```python
from build123d import *

# Parameters (mm, degrees)
F0_W     = 26.5
F0_H     = 53
F1_DEPTH = 11
F2_R     = 5.75
F3_DEPTH = 120
F4_W     = 18
F4_H     = 11
F5_DEPTH = 25


with BuildPart() as f1:
    # F0 (on Top) → F1 (new body)
    with BuildSketch(Plane.XY):
        Rectangle(F0_W, F0_H)
    extrude(amount=F1_DEPTH)

    # F2 (on face) → F3 (join)
    with BuildSketch(Plane(origin=(0, 26.5, 0), x_dir=(-1, 0, 0), z_dir=(0, 1, 0))):
        with Locations((-5.25, 5.5)):
            Circle(F2_R)
    extrude(amount=F3_DEPTH)

    # F4 (on face) → F5 (join)
    with BuildSketch(Plane.XZ.offset(26.5)):
        with Locations((0, 5.5)):
            Rectangle(F4_W, F4_H)
    extrude(amount=F5_DEPTH)


solid = f1.part
```
Design review of the part built by this model. Coordinates are the model's own, in mm. A direction names the side the tool comes from. Round coordinates to 2 decimals unless told otherwise and drop trailing zeros. Write each loop counter-clockwise with the first axis right and the second up, starting at its lowest first coordinate (ties: lowest second). Pieces come first, ordered by that corner, then holes. Notation, with made-up numbers: (48, -18.5) -> (58, -18.5) arc R24 cw to (58, 12.5) -> close; hole circle Ø6 at (-27, 22). An arc over 180 degrees is marked (long way). Write item = value, one per line. Start each with the question number.
1) Wall thickness on probe 1 along X at (y, z) = (111.5, 6); probe 2 along Z at (x, y) = (-1.25, -27.5); probe 3 along Y at (x, z) = (-2.25, 9): over which ranges is each line inside the solid? List them lowest first. Write a range as from..to.
2) Take a section at A-A, the plane z = 5.5. State the section outline as (x, y) points.
3) Take a section at D-D, the plane x = -5. State the section outline as (y, z) points, plus the area to 3 significant figures.
4) Take a section at C-C, the plane y = -33. State the section outline as (x, z) points, plus the area to 3 significant figures.
5) Take a section at B-B, the plane x = 5.25. State the section outline as (y, z) points, plus the area to 3 significant figures.
6) Clearance check with flat-ended pins moving along their axes: pin 1 (1 mm diameter, centred on x = 10, y = 39, fed in from -Z); pin 2 (3 mm diameter, centred on x = 2.5, y = 36, fed in from -Z); pin 3 (5.5 mm diameter, centred on y = -37.5, z = 5, fed in from +X). State where each tip first meets the part, or that it passes through.
7) Tool access review of faces 1 (the face through (6, 85.7, 11.2)), 2 (the face through (-11, -26.5, 5)), 3 (the face through (11, -26.5, 5)): name each direction out of +Z, -Z, +X, -X, +Y, -Y from which nothing blocks a thin tool from reaching the whole face with its end or side.
Results list:
q1.probe_1 = -0.48..10.98
q1.probe_2 = 0..11
q1.probe_3 = -51.5..26.5
q2.outline = (-13.25, -26.5) -> (-9, -26.5) -> (-9, -51.5) -> (9, -51.5) -> (9, -26.5) -> (13.25, -26.5) -> (13.25, 26.5) -> (11, 26.5) -> (11, 146.5) -> (-0.5, 146.5) -> (-0.5, 26.5) -> (-13.25, 26.5) -> close
q3.outline = (-51.5, 0) -> (26.5, 0) -> (26.5, 11) -> (-51.5, 11) -> close
q3.area = 858 mm²
q4.outline = (-9, 0) -> (9, 0) -> (9, 11) -> (-9, 11) -> close
q4.area = 198 mm²
q5.outline = (-51.5, 0) -> (26.5, 0) -> (26.5, -0.25) -> (146.5, -0.25) -> (146.5, 11.25) -> (26.5, 11.25) -> (26.5, 11) -> (-51.5, 11) -> close
q5.area = 2,240 mm²
q6.pin_1 = 1.63
q6.pin_2 = -0.11
q6.pin_3 = 9
q7.face_1 = +Y
q7.face_2 = +Z, -Z, -X, -Y
q7.face_3 = +Z, -Z, +X, -Y
